from build123d import *

# Parameters (mm, degrees)
SKETCH_1_W          = 20
SKETCH_1_H          = 10
SKETCH_1_R          = 1.5
EXTRUDE_1_DEPTH     = 54
EXTRUDE_2_DEPTH     = 54
FILLET_1_R          = 3
SKETCH_4_R          = 1.5
CUT_EXTRUDE_2_DEPTH = 16


with BuildPart() as part:
    # 草图1 → 凸台-拉伸1 (new body)
    with BuildSketch(Plane.XY):
        Rectangle(SKETCH_1_W, SKETCH_1_H)
        with Locations((-6, 0)):
            Circle(SKETCH_1_R, mode=Mode.SUBTRACT)
        with Locations((6, 0)):
            Circle(SKETCH_1_R, mode=Mode.SUBTRACT)
    extrude(amount=EXTRUDE_1_DEPTH)

    # 草图2 → 凸台-拉伸2 (add)
    with BuildSketch(Plane(origin=(0, 0, 0), x_dir=(-1, 0, 0), z_dir=(0, 0, -1))):
        Polygon((-26.016199375, 3.045755137), (-10, 5), (-10, -5), (10, -5), (-13.936339886, -9.975800078), align=None)
    extrude(amount=-EXTRUDE_2_DEPTH)

    # 圆角1
    fillet_1_edges = [part.edges().sort_by_distance(p)[0] for p in [
        (26.016199375, 3.045755137, 27),
        (13.936339886, -9.975800078, 27),
        (-10, -5, 27),
        (-10, 5, 27),
        (10, 5, 27),
    ]]
    fillet(fillet_1_edges, radius=FILLET_1_R)

    # 草图4 → 切除-拉伸2 (cut)
    with BuildSketch(Plane.XY.offset(54)):
        with BuildLine():
            Line((9.817651049, 5), (0, 5))
            Line((0, 5), (0, -7.078763964))
            Line((0, -7.078763964), (12.278210403, -9.631114097))
            ThreePointArc((12.278210403, -9.631114097), (13.801017817, -9.551847513), (15.088142689, -8.734207508))
            Line((15.088142689, -8.734207508), (22.02094679, -1.260950763))
            ThreePointArc((22.02094679, -1.260950763), (22.638947239, 1.810129636), (20.184946376, 3.757265774))
            Line((20.184946376, 3.757265774), (10.181006508, 4.977914171))
            ThreePointArc((10.181006508, 4.977914171), (9.99966408, 4.994473452), (9.817651049, 5))
        make_face()
        with Locations((6, 0)):
            Circle(SKETCH_4_R, mode=Mode.SUBTRACT)
    extrude(amount=-CUT_EXTRUDE_2_DEPTH, mode=Mode.SUBTRACT)


solid = part.part
Check sheet for the modelled part. Datum: model origin and axes. Units: mm. A direction names the side the tool comes from. Round coordinates to 2 decimals unless told otherwise and drop trailing zeros. Order: outer loops, then holes, each group sorted by start corner. A loop starts at its lowest first (then second) coordinate and runs counter-clockwise, first axis right, second up. Notation, with made-up numbers: M 24.25,52 L 47.25,52 A34 cw 47.25,91 Z; hole C -5.5,74 d1. An arc over 180 degrees is marked long. One line per item, written item: value. Start each with the question number.
1. Section check C-C on y = 0. Enter the section's corners in (x, z).
2. Section check A-A on z = 10. Enter the section's corners in (x, y), and give its area (3 significant figures).
3. Gauge pin test, flat ends, axial feed: P1, Ø1, axis at x = 17.5, z = 24.5, coming from the -Y side; P2, Ø10, axis at x = 0, z = 7.5, coming from the -Y side; P3, Ø3.5, axis at x = 6, y = 0, coming from the +Z side. Record the tip position at first contact, or that the pin passes through.
4. Section check B-B on x = -6. Enter the section's corners in (y, z), and give its area (3 significant figures).
5. Release check for a two-part mould opening along X. For faces 3 (the flat face through (-10, 0, 27)), 4 (the flat face through (6, -2, 0)), 5 (the cylindrical face through (-7.2, -0.9, 26.6)), 6 (the cylindrical face through (13.822, -9.545, 19.266)) record: released by +X, released by -X, zero draft, split by the parting line, or undercut.
6. Access from +Z, -Z, +X, -X, +Y, -Y to the whole of each face (thin tool, end or side, straight path). Record for faces 1 (the cylindrical face through (-9.1, 4.14, 27.38)), 2 (the flat face through (11, -2, 38)).
7. Section check D-D on z = 45.5. Enter the section's corners in (x, y), and give its area (3 significant figures).
8. Scan lines: line 1 along Z through (x, y) = (2.5, -2.5); line 2 along X through (y, z) = (0.25, 43); line 3 along Y through (x, z) = (6, 21). Record each from-to range of solid material in increasing order.
Results found:
1. outline: M -10,0 L -7.5,0 L -7.5,54 L -10,54 Z; M -4.5,0 L 4.5,0 L 4.5,38 L 0,38 L 0,54 L -4.5,54 Z; M 7.5,0 L 22.72,0 L 22.72,38 L 7.5,38 Z
2. outline: M -10,-2.56 A3 ccw -7.61,-5.5 L 12.28,-9.63 A3 ccw 15.09,-8.73 L 22.02,-1.26 A3 ccw 20.18,3.76 L 10.18,4.98 A3 ccw 9.82,5 L -7,5 A3 ccw -10,2 Z; hole C -6,0 d3; hole C 6,0 d3
2. area: 360 mm^2
3. P1: y = -6.67
3. P2: y = -8.12
3. P3: z = 38
4. outline: M -5.83,0 L -1.5,0 L -1.5,54 L -5.83,54 Z; M 1.5,0 L 5,0 L 5,54 L 1.5,54 Z
4. area: 423 mm^2
5. face 3: released by -X
5. face 4: zero draft
5. face 5: undercut
5. face 6: split by the parting line
6. face 1: +Z, -Z, -X, +Y
6. face 2: +Z, +X, +Y, -Y
7. outline: M -10,-2.56 A3 ccw -7.61,-5.5 L 0,-7.08 L 0,5 L -7,5 A3 ccw -10,2 Z; hole C -6,0 d3
7. area: 100 mm^2
8. line 1: 0 to 38
8. line 2: -10 to -7.48, -4.52 to 0
8. line 3: -8.33 to -1.5, 1.5 to 5
